Read the model definition and answer for the solid it produces. Units are mm, in the model's axes. Face numbers are marked on the shaded views. Round coordinates to 2 decimals unless told otherwise and drop trailing zeros. Write each loop counter-clockwise with the first axis right and the second up, starting at its lowest first coordinate (ties: lowest second). Pieces come first, ordered by that corner, then holes. Notation, with made-up numbers: (-36, 21) - (-7, 21) arc R12 cw to (-7, 41) - close; hole circle Ø3 at (82, -25.75). An arc over 180 degrees is marked (long way). Use one line per item in the form item = value. Start each with the question number.
1) The part is cut by section D-D, the plane y = 16. Give the vertices of the cut face in (x, z).
2) For a pull along Y with two mould halves and no side action, classify the marked faces 1, 2 and 3 as released by +Y, released by -Y, zero draft, split by the parting line, or undercut.
3) The part is cut by section B-B, the plane y = 0. Give the vertices of the cut face in (x, z), plus the area to 3 significant figures.
4) The part is cut by section A-A, the plane z = 11.5. Give the vertices of the cut face in (x, y), plus the area to 3 significant figures.
5) Each of these flat-tipped pins is pushed along its axis until it touches: pin 1 (2 mm diameter, centred on x = -2, z = 10.5, fed in from -Y); pin 2 (10 mm diameter, centred on y = -7.5, z = 8.5, fed in from +X); pin 3 (2 mm diameter, centred on x = -12.5, y = 8.5, fed in from +Z). Where does it stop, or does it pass through?
6) The part is cut by section C-C, the plane x = 19. Give the vertices of the cut face in (y, z).
7) Consider line 1 along X through (y, z) = (-2.5, 4); line 2 along Y through (x, z) = (27, 15.25); line 3 along Y through (x, z) = (-5.5, 12). Determine where each line is inside the solid, lowest interval first. Write a range as from..to.
from build123d import *

# Parameters (mm, degrees)
F1_ANGLE = 180
F3_ANGLE = 180
F5_ANGLE = 180


with BuildPart() as f1:
    # F0 (on Top) → F1 (revolve)
    with BuildSketch(Plane.XY):
        Polygon((22.25, -22.25), (22.25, 0), (17.25, 0), (17.25, -17.25), (-17.25, -17.25), (-17.25, 0), (-22.25, 0), (-22.25, -22.25), align=None)
    revolve(axis=Axis((4.6253763139, 0, 0), (-1, 0, 0)), revolution_arc=F1_ANGLE)

    # F2 (on face) → F3 (revolve)
    with BuildSketch(Plane.YZ.offset(22.25)):
        with BuildLine():
            ThreePointArc((0, 22.25), (-15.7331258814, 15.7331258814), (-22.25, 0))
            Line((-22.25, 0), (-17.25, 0))
            ThreePointArc((-17.25, 0), (-12.1975919755, 12.1975919755), (0, 17.25))
            Line((0, 17.25), (0, 22.25))
        make_face()
    revolve(axis=Axis((22.25, 0, 10.080948472), (0, 0, 1)), revolution_arc=F3_ANGLE)

    # F4 (on face) → F5 (revolve)
    with BuildSketch(Plane(origin=(-22.25, 0, 0), x_dir=(0, -1, 0), z_dir=(-1, 0, 0))):
        with BuildLine():
            ThreePointArc((0, 22.25), (-15.7331258814, 15.7331258814), (-22.25, 0))
            Line((-22.25, 0), (-17.6879018545, 0))
            ThreePointArc((-17.6879018545, 0), (-12.5072353463, 12.5072353463), (0, 17.6879018545))
            Line((0, 17.6879018545), (0, 22.25))
        make_face()
    revolve(axis=Axis((-22.25, 0, 6.120197475), (0, 0, 1)), revolution_arc=F5_ANGLE)


solid = f1.part
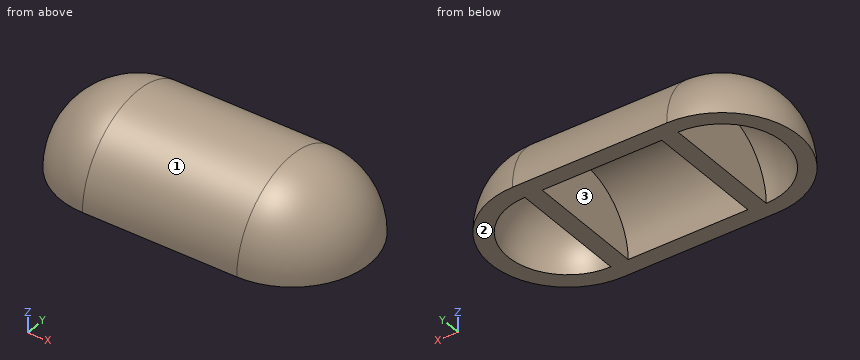
Geometry results:
q1.outline = (-37.71, 0) - (-29.79, 0) arc R7.54 cw to (-22.25, 7.54) - (-22.25, 0) - (-17.25, 0) - (-17.25, 6.45) - (17.25, 6.45) - (17.25, 0) - (22.25, 0) - (22.25, 6.45) arc R6.45 cw to (28.7, 0) - (37.71, 0) arc R15.46 ccw to (22.25, 15.46) - (-22.25, 15.46) arc R15.46 ccw to start
q2.face_1 = split by the parting line
q2.face_2 = zero draft
q2.face_3 = undercut
q3.outline = (-44.5, 0) - (-39.94, 0) arc R17.69 cw to (-22.25, 17.69) - (-22.25, 0) - (-17.25, 0) - (-17.25, 17.25) - (17.25, 17.25) - (17.25, 0) - (22.25, 0) - (22.25, 17.25) arc R17.25 cw to (39.5, 0) - (44.5, 0) arc R22.25 ccw to (22.25, 22.25) - (-22.25, 22.25) arc R22.25 ccw to start
q3.area = 693 mm2
q4.outline = (-22.25, -19.05) - (22.25, -19.05) arc R19.05 ccw to (22.25, 19.05) - (-22.25, 19.05) arc R19.05 ccw to start; hole (-22.25, -13.44) - (-22.25, 13.44) arc R13.44 ccw to start; hole (-17.25, -12.86) - (17.25, -12.86) - (17.25, 12.86) - (-17.25, 12.86) - close; hole (22.25, -12.86) arc R12.86 ccw to (22.25, 12.86) - close
q4.area = 1,400 mm2
q5.pin_1 = -20.12
q5.pin_2 = 43.58
q5.pin_3 = 20.95
q6.outline = (-22.25, 0) - (22.25, 0) arc R22.25 ccw to start
q7.line_1 = -43.99..-39.3, -22.25..-17.25, 17.25..22.25, 38.84..43.99
q7.line_2 = -15.49..-6.51, 6.51..15.49
q7.line_3 = -18.74..-12.39, 12.39..18.74
